```python
from build123d import *

# Parameters (mm, degrees)
SKETCH_3_W             = 7.8
SKETCH_3_H             = 23.4
SKETCH_3_W_2           = 8
SKETCH_3_H_2           = 7.8
SKETCH_3_W_3           = 0.1
EXTRUDE_1_DEPTH        = 7.4
CUT_EXTRUDE_1_REACH    = 22.97
SKETCH_4_R             = 2.5
SKETCH_4_3_R           = 3.15
SKETCH_4_3_R_2         = 2.5
CUT_EXTRUDE_2_DEPTH    = 1
CUT_EXTRUDE_START      = -6.8
SKETCH_4_4_R           = 3.15
SKETCH_4_4_R_2         = 2.5
CUT_EXTRUDE_3_DEPTH    = 1
SKETCH_5_R             = 2.5
CUT_EXTRUDE_4_DEPTH    = 35.187132082
SKETCH_5_3_R           = 3.15
SKETCH_5_3_R_2         = 2.5
CUT_EXTRUDE_5_DEPTH    = 1
SKETCH_5_4_R           = 3.15
SKETCH_5_4_R_2         = 2.5
CUT_EXTRUDE_6_DEPTH    = 1
CUT_EXTRUDE_START_2    = -16
SKETCH_5_5_R           = 3.15
SKETCH_5_5_R_2         = 2.5
CUT_EXTRUDE_7_DEPTH    = 1
CUT_EXTRUDE_START_3    = -22.8
SKETCH_5_6_R           = 3.15
SKETCH_5_6_R_2         = 2.5
CUT_EXTRUDE_8_DEPTH    = 1
PATTERN_LINEAR_1_COUNT = 2
PATTERN_LINEAR_1_PITCH = 8
CUT_EXTRUDE_9_DEPTH    = 2
CUT_EXTRUDE_START_4    = -5.8
CUT_EXTRUDE_10_DEPTH   = 2
CUT_EXTRUDE_11_DEPTH   = 2
CUT_EXTRUDE_START_5    = -21.8
CUT_EXTRUDE_12_DEPTH   = 2
PATTERN_LINEAR_2_COUNT = 2
PATTERN_LINEAR_2_PITCH = 8
FILLET_1_R             = 3.5


with BuildPart() as part:
    # 草图3 → 凸台-拉伸1 (new body)
    with BuildSketch(Plane(origin=(0, 0, 0), x_dir=(0, 0, -1), z_dir=(1, 0, 0))):
        with Locations((-8, 11.7)):
            Rectangle(SKETCH_3_W, SKETCH_3_H)
        with Locations((8, 11.7)):
            Rectangle(SKETCH_3_W, SKETCH_3_H)
        with Locations((0, 3.9)):
            Rectangle(SKETCH_3_W_2, SKETCH_3_H_2)
        with Locations((-4.05, 3.9)):
            Rectangle(SKETCH_3_W_3, SKETCH_3_H_2)
        with Locations((4.05, 3.9)):
            Rectangle(SKETCH_3_W_3, SKETCH_3_H_2)
    extrude(amount=EXTRUDE_1_DEPTH)

    # 草图4 → 切除-拉伸1 (cut, up to next)
    with BuildSketch(Plane(origin=(0, 7.8, 0), x_dir=(1, 0, 0), z_dir=(0, 1, 0)), mode=Mode.PRIVATE) as cut_extrude_1_sk1:
        with Locations(Location((3.7, 0, 0), (0, 0, 270))):
            Circle(SKETCH_4_R)
    cut_extrude_1_tool1 = extrude(cut_extrude_1_sk1.sketch, amount=-CUT_EXTRUDE_1_REACH, mode=Mode.PRIVATE) & part.part
    add(cut_extrude_1_tool1.solids().sort_by_distance((3.7, 7.8, 0))[0], mode=Mode.SUBTRACT)

    # 草图4<3> → 切除-拉伸2 (cut)
    with BuildSketch(Plane(origin=(0, 7.8, 0), x_dir=(1, 0, 0), z_dir=(0, 1, 0))):
        with Locations(Location((3.7, 0, 0), (0, 0, 270))):
            Circle(SKETCH_4_3_R)
        with Locations(Location((3.7, 0, 0), (0, 0, 270))):
            Circle(SKETCH_4_3_R_2, mode=Mode.SUBTRACT)
    extrude(amount=-CUT_EXTRUDE_2_DEPTH, mode=Mode.SUBTRACT)

    # 草图4<4> → 切除-拉伸3 (cut)
    with BuildSketch(Plane(origin=(0, 7.8, 0), x_dir=(1, 0, 0), z_dir=(0, 1, 0)).offset(CUT_EXTRUDE_START)):
        with Locations(Location((3.7, 0, 0), (0, 0, 270))):
            Circle(SKETCH_4_4_R)
        with Locations(Location((3.7, 0, 0), (0, 0, 270))):
            Circle(SKETCH_4_4_R_2, mode=Mode.SUBTRACT)
    extrude(amount=-CUT_EXTRUDE_3_DEPTH, mode=Mode.SUBTRACT)

    # 草图5 → 切除-拉伸4 (cut, through all)
    with BuildSketch(Plane(origin=(0, 0, -11.9), x_dir=(-1, 0, 0), z_dir=(0, 0, -1))):
        with Locations((-3.7, 11.7)):
            Circle(SKETCH_5_R)
    cut_extrude_4 = extrude(amount=-CUT_EXTRUDE_4_DEPTH, mode=Mode.SUBTRACT)

    # 草图5<3> → 切除-拉伸5 (cut)
    with BuildSketch(Plane(origin=(0, 0, -11.9), x_dir=(-1, 0, 0), z_dir=(0, 0, -1))):
        with Locations((-3.7, 11.7)):
            Circle(SKETCH_5_3_R)
        with Locations((-3.7, 11.7)):
            Circle(SKETCH_5_3_R_2, mode=Mode.SUBTRACT)
    cut_extrude_5 = extrude(amount=-CUT_EXTRUDE_5_DEPTH, mode=Mode.SUBTRACT)

    # 草图5<4> → 切除-拉伸6 (cut)
    with BuildSketch(Plane(origin=(0, 0, -11.9), x_dir=(-1, 0, 0), z_dir=(0, 0, -1)).offset(CUT_EXTRUDE_START)):
        with Locations((-3.7, 11.7)):
            Circle(SKETCH_5_4_R)
        with Locations((-3.7, 11.7)):
            Circle(SKETCH_5_4_R_2, mode=Mode.SUBTRACT)
    cut_extrude_6 = extrude(amount=-CUT_EXTRUDE_6_DEPTH, mode=Mode.SUBTRACT)

    # 草图5<5> → 切除-拉伸7 (cut)
    with BuildSketch(Plane(origin=(0, 0, -11.9), x_dir=(-1, 0, 0), z_dir=(0, 0, -1)).offset(CUT_EXTRUDE_START_2)):
        with Locations((-3.7, 11.7)):
            Circle(SKETCH_5_5_R)
        with Locations((-3.7, 11.7)):
            Circle(SKETCH_5_5_R_2, mode=Mode.SUBTRACT)
    cut_extrude_7 = extrude(amount=-CUT_EXTRUDE_7_DEPTH, mode=Mode.SUBTRACT)

    # 草图5<6> → 切除-拉伸8 (cut)
    with BuildSketch(Plane(origin=(0, 0, -11.9), x_dir=(-1, 0, 0), z_dir=(0, 0, -1)).offset(CUT_EXTRUDE_START_3)):
        with Locations((-3.7, 11.7)):
            Circle(SKETCH_5_6_R)
        with Locations((-3.7, 11.7)):
            Circle(SKETCH_5_6_R_2, mode=Mode.SUBTRACT)
    cut_extrude_8 = extrude(amount=-CUT_EXTRUDE_8_DEPTH, mode=Mode.SUBTRACT)

    # 阵列(线性)1: 切除-拉伸4, 切除-拉伸5, 切除-拉伸6, 切除-拉伸7, 切除-拉伸8 ×2
    with Locations(*[(0, i * PATTERN_LINEAR_1_PITCH, 0) for i in range(1, PATTERN_LINEAR_1_COUNT)]):
        add(cut_extrude_4, mode=Mode.SUBTRACT)
        add(cut_extrude_5, mode=Mode.SUBTRACT)
        add(cut_extrude_6, mode=Mode.SUBTRACT)
        add(cut_extrude_7, mode=Mode.SUBTRACT)
        add(cut_extrude_8, mode=Mode.SUBTRACT)

    # 草图6 → 切除-拉伸9 (cut)
    with BuildSketch(Plane(origin=(0, 0, -11.9), x_dir=(-1, 0, 0), z_dir=(0, 0, -1))):
        with BuildLine():
            ThreePointArc((-6.525, 14.089429848), (-3.7, 15.4), (-0.875, 14.089429848))
            Line((-0.875, 14.089429848), (-0.875, 17.310570152))
            ThreePointArc((-0.875, 17.310570152), (-3.7, 16), (-6.525, 17.310570152))
            Line((-6.525, 17.310570152), (-6.525, 14.089429848))
        make_face()
    cut_extrude_9 = extrude(amount=-CUT_EXTRUDE_9_DEPTH, mode=Mode.SUBTRACT)

    # 草图6<3> → 切除-拉伸10 (cut)
    with BuildSketch(Plane(origin=(0, 0, -11.9), x_dir=(-1, 0, 0), z_dir=(0, 0, -1)).offset(CUT_EXTRUDE_START_4)):
        with BuildLine():
            ThreePointArc((-6.525, 14.089429848), (-3.7, 15.4), (-0.875, 14.089429848))
            Line((-0.875, 14.089429848), (-0.875, 17.310570152))
            ThreePointArc((-0.875, 17.310570152), (-3.7, 16), (-6.525, 17.310570152))
            Line((-6.525, 17.310570152), (-6.525, 14.089429848))
        make_face()
    cut_extrude_10 = extrude(amount=-CUT_EXTRUDE_10_DEPTH, mode=Mode.SUBTRACT)

    # 草图6<4> → 切除-拉伸11 (cut)
    with BuildSketch(Plane(origin=(0, 0, -11.9), x_dir=(-1, 0, 0), z_dir=(0, 0, -1)).offset(CUT_EXTRUDE_START_2)):
        with BuildLine():
            ThreePointArc((-6.525, 14.089429848), (-3.7, 15.4), (-0.875, 14.089429848))
            Line((-0.875, 14.089429848), (-0.875, 17.310570152))
            ThreePointArc((-0.875, 17.310570152), (-3.7, 16), (-6.525, 17.310570152))
            Line((-6.525, 17.310570152), (-6.525, 14.089429848))
        make_face()
    cut_extrude_11 = extrude(amount=-CUT_EXTRUDE_11_DEPTH, mode=Mode.SUBTRACT)

    # 草图6<5> → 切除-拉伸12 (cut)
    with BuildSketch(Plane(origin=(0, 0, -11.9), x_dir=(-1, 0, 0), z_dir=(0, 0, -1)).offset(CUT_EXTRUDE_START_5)):
        with BuildLine():
            ThreePointArc((-6.525, 14.089429848), (-3.7, 15.4), (-0.875, 14.089429848))
            Line((-0.875, 14.089429848), (-0.875, 17.310570152))
            ThreePointArc((-0.875, 17.310570152), (-3.7, 16), (-6.525, 17.310570152))
            Line((-6.525, 17.310570152), (-6.525, 14.089429848))
        make_face()
    cut_extrude_12 = extrude(amount=-CUT_EXTRUDE_12_DEPTH, mode=Mode.SUBTRACT)

    # 阵列(线性)2: 切除-拉伸9, 切除-拉伸10, 切除-拉伸11, 切除-拉伸12 ×2
    with Locations(*[(0, -i * PATTERN_LINEAR_2_PITCH, 0) for i in range(1, PATTERN_LINEAR_2_COUNT)]):
        add(cut_extrude_9, mode=Mode.SUBTRACT)
        add(cut_extrude_10, mode=Mode.SUBTRACT)
        add(cut_extrude_11, mode=Mode.SUBTRACT)
        add(cut_extrude_12, mode=Mode.SUBTRACT)

    # 圆角1
    fillet_1_edges = [part.edges().sort_by_distance(p)[0] for p in [
        (7.4, 23.4, -8),
        (0, 23.4, 8),
        (0, 23.4, -8),
        (3.7, 0, -11.9),
        (3.7, 0, 11.9),
        (7.4, 23.4, 8),
    ]]
    fillet(fillet_1_edges, radius=FILLET_1_R)


solid = part.part
```
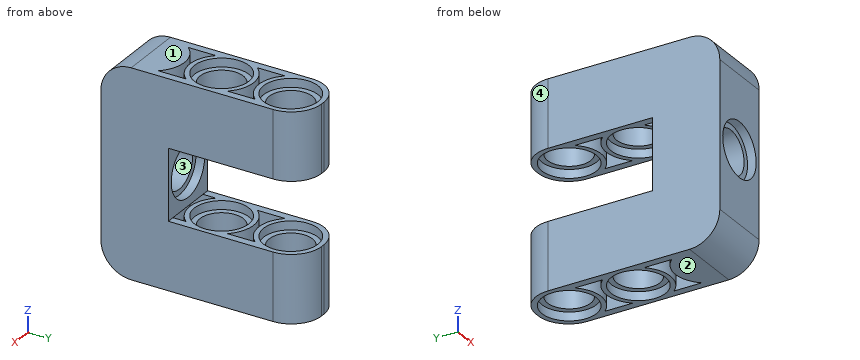
Check sheet for the modelled part. Datum: model origin and axes. Units: mm. Face numbers are marked on the shaded views. Coordinates: 2 decimals unless noted, no trailing zeros. Write each loop counter-clockwise with the first axis right and the second up, starting at its lowest first coordinate (ties: lowest second). Pieces come first, ordered by that corner, then holes. Notation, with made-up numbers: M 41.5,61.5 L 99.5,61.5 A18 cw 99.5,85.5 Z; hole C -1,38.5 d11. An arc over 180 degrees is marked long. Write item = value, one per line. Start each with the question number.
1. Sectioned sample at A-A (z = 0). Record the cut outline in (x, y), then the cut area to 3 significant figures.
2. Mould release check, pull along Z, two halves, no side actions. Record for the marked faces 1, 2, 3 and 4: pulls with the +Z half, pulls with the -Z half, needs draft (parallel to the pull), parting line crosses it, or undercut.
3. Thickness scan on probe 1 along Z at (x, y) = (7, 19.5); probe 2 along Z at (x, y) = (5.75, 16); probe 3 along Y at (x, z) = (6, 7). Record the ranges inside material, lowest first.
4. Sectioned sample at B-B (y = 11.7). State how many separate pieces and enclosed holes the cut face has, then the cut area to 3 significant figures.
5. Sectioned sample at C-C (z = -5.5). Record the cut outline in (x, y) (3 decimals).
The answers:
q1.outline = M 0,0 L 0.55,0 L 0.55,1 L 1.2,1 L 1.2,6.8 L 0.55,6.8 L 0.55,7.8 L 0,7.8 Z; M 6.2,1 L 6.85,1 L 6.85,0 L 7.4,0 L 7.4,7.8 L 6.85,7.8 L 6.85,6.8 L 6.2,6.8 Z
q1.area = 16.1 mm²
q2.face_1 = pulls with the +Z half
q2.face_2 = pulls with the -Z half
q2.face_3 = undercut
q2.face_4 = needs draft
q3.probe_1 = -11.9 to -4.1, 4.1 to 11.9
q3.probe_2 = -9.9 to -6.1, 6.1 to 9.9
q3.probe_3 = 0 to 10.72, 12.68 to 18.72, 20.68 to 22.7
q4.separate_pieces = 4
q4.enclosed_holes = 0
q4.area = 32.2 mm²
q5.outline = M 0,0 L 7.4,0 L 7.4,19.9 A3.5 ccw 3.9,23.4 L 3.5,23.4 A3.5 ccw 0,19.9 Z; hole M 0.875,6.089 A3.7 cw 6.525,6.089 L 6.525,9.311 A3.7 cw 0.875,9.311 Z; hole M 0.875,14.089 A3.7 cw 6.525,14.089 L 6.525,17.311 A3.7 cw 0.875,17.311 Z; hole C 3.7,11.7 d5; hole C 3.7,19.7 d5
